from build123d import *

# Parameters (mm, degrees)
CHAMFER1_SIZE = 1


with BuildPart() as part:
    # Sketch1 → Revolve1 (revolve)
    with BuildSketch(Plane(origin=(0, 0, 0), x_dir=(0, 0, -1), z_dir=(1, 0, 0)), mode=Mode.PRIVATE) as revolve1_sk:
        Polygon((0, 0), (0, 2.5), (8.5, 2.5), (8.5, 11), (11.5, 11), (11.5, 5), (15.5, 5), (15.5, 3), (21, 3), (21, 0), align=None)
    revolve(revolve1_sk.sketch.rotate(Axis((0, 0, 41.619499546), (0, 0, -1)), 90), axis=Axis((0, 0, 41.619499546), (0, 0, -1)))

    # Chamfer1
    chamfer1_edges = [part.edges().sort_by_distance(p)[0] for p in [
        (-2.5, 0, 0),
        (-3, 0, -21),
    ]]
    chamfer(chamfer1_edges, length=CHAMFER1_SIZE)


solid = part.part
Could you check a few things on this model? Use its own coordinates, in mm. A direction names the side the tool comes from. Give positions to 0.01 mm unless a question says otherwise; leave off trailing zeros. Order: outer loops, then holes, each group sorted by start corner. A loop starts at its lowest first (then second) coordinate and runs counter-clockwise, first axis right, second up.
Item 1: For faces 1 (the face through (-2.5, -0.1, -4.8)), 2 (the face through (-2.38, 10.74, -10.02)), 3 (the face through (3.3, -0.1, -15.5)), which set-ups out of +Z, -Z, +X, -X, +Y, -Y let a thin tool reach every point of the face, with its end or its side?
Item 2: If we mould it in two halves opening along Z, with no side actions, what happens to faces 4 (the face through (0, 0, -21)), 5 (the face through (0, 0, 0)), 6 (the face through (-5, 0, -14))? For each: pulls with the +Z half, pulls with the -Z half, needs draft (parallel to the pull), parting line crosses it, or undercut.
Item 3: If we section it at D-D, the plane x = -4.5: Write out the boundary of the cut face in (y, z).
Item 4: If we section it at C-C, the plane z = -1.5: Write out the boundary of the cut face in (x, y).
Item 5: I need wall thicknesses on line 1 (Z direction, x = -8.5, y = 6.25); line 2 (Y direction, x = 0, z = -2.25); line 3 (Y direction, x = -3, z = -10). Which ranges of each line are inside material? Lowest first, please.
Item 6: I'm going to push flat-ended pins straight in: pin 1 (3 mm diameter, centred on y = -8.5, z = -10, fed in from -X); pin 2 (1 mm diameter, centred on y = -8.5, z = -11.5, fed in from -X); pin 3 (12 mm diameter, centred on x = 6, z = -18, fed in from +Y). Where does each tip first touch, or does it pass through?
Item 7: If we section it at A-A, the plane x = 0: Write out the boundary of the cut face in (y, z), plus the area to 4 significant figures.
Values:
1. face 1: +Z
1. face 2: +Z, -Z
1. face 3: -Z
2. face 4: pulls with the -Z half
2. face 5: pulls with the +Z half
2. face 6: needs draft
3. outline: (-10.04, -11.5) - (-2.18, -11.5) - (-2.18, -15.5) - (2.18, -15.5) - (2.18, -11.5) - (10.04, -11.5) - (10.04, -8.5) - (-10.04, -8.5) - close
4. outline: circle Ø5 at (0, 0)
5. line 1: z = -11.5 to -8.5
5. line 2: y = -2.5 to 2.5
5. line 3: y = -10.58 to 10.58
6. pin 1: stops at x = -8.49
6. pin 2: stops at x = -7.55
6. pin 3: stops at y = 4.97
7. outline: (-11, -11.5) - (-5, -11.5) - (-5, -15.5) - (-3, -15.5) - (-3, -20) - (-2, -21) - (2, -21) - (3, -20) - (3, -15.5) - (5, -15.5) - (5, -11.5) - (11, -11.5) - (11, -8.5) - (2.5, -8.5) - (2.5, -1) - (1.5, 0) - (-1.5, 0) - (-2.5, -1) - (-2.5, -8.5) - (-11, -8.5) - close
7. area: 179.5 mm2
